CAD build for the part. Positions are in the model's coordinates, mm. Round coordinates to 2 decimals unless told otherwise and drop trailing zeros. Write each loop counter-clockwise with the first axis right and the second up, starting at its lowest first coordinate (ties: lowest second). Pieces come first, ordered by that corner, then holes. Notation, with made-up numbers: (66, -32) - (87, -32) arc R26 cw to (87, -15) - close; hole circle Ø11 at (88.25, -27). An arc over 180 degrees is marked (long way). Put each result on its own line as item: value. Start each with the question number.
Item 1: Pin check, flat tips, straight feed: pin 1 Ø2.5 at (y, z) = (-15, 120) entering from -X; pin 2 Ø5 at (x, z) = (5, 95) entering from -Y. Stop position of each tip, or through.
Item 2: Cut at A-A (x = 11). Give the cut face in (y, z), and give its area (3 significant figures).
Item 3: Drill centre lines: line 1 (X direction, y = -18.9, z = 55) (3 decimals); line 2 (X direction, y = -6.75, z = 173); line 3 (Y direction, x = 11, z = 27). Where is each one in solid material? Low to high. Write a range as from..to.
Item 4: Mould opens along X. For faces 1 (the cylindrical face through (5.473, -0.74, 191.502)), 2 (the cylindrical face through (0.74, -4.659, 18.462)), 3 (the cylindrical face through (14.397, -19.24, 121.455)) say: released by +X, released by -X, zero draft, split by the parting line, or undercut.
Item 5: Cut at B-B (z = 106). Give the cut face in (x, y), and give its area (3 significant figures).
Item 6: Cut at C-C (z = 76.5). Give the cut face in (x, y), and give its area (3 significant figures).
```python
from build123d import *

# Parameters (mm, degrees)
SKETCH_1_W          = 20
SKETCH_1_H          = 20
SKETCH_1_W_2        = 17
SKETCH_1_H_2        = 17
EXTRUDE_1_DEPTH     = 205
SKETCH_2_R          = 2.7
SKETCH_2_R_2        = 1.575
CUT_EXTRUDE_1_DEPTH = 207.942020866
SKETCH_3_R          = 1.575
CUT_EXTRUDE_2_DEPTH = 207.942020866


with BuildPart() as part:
    # 草图1 → 拉伸-薄壁1 (new body)
    with BuildSketch(Plane.XY):
        with Locations((10, -10)):
            Rectangle(SKETCH_1_W, SKETCH_1_H)
        with Locations((10, -10)):
            Rectangle(SKETCH_1_W_2, SKETCH_1_H_2, mode=Mode.SUBTRACT)
    extrude(amount=EXTRUDE_1_DEPTH)

    # 草图2 → 切除-拉伸1 (cut, through all)
    with BuildSketch(Plane.ZY):
        with Locations(Location((106, -15, 0), (0, 0, 270))):
            Circle(SKETCH_2_R)
        with Locations(Location((180, -5, 0), (0, 0, 270))):
            Circle(SKETCH_2_R_2)
        with Locations(Location((180, -15, 0), (0, 0, 270))):
            Circle(SKETCH_2_R_2)
        with Locations(Location((170, -15, 0), (0, 0, 270))):
            Circle(SKETCH_2_R_2)
        with Locations(Location((170, -5, 0), (0, 0, 270))):
            Circle(SKETCH_2_R_2)
        with Locations(Location((120, -5, 0), (0, 0, 270))):
            Circle(SKETCH_2_R_2)
        with Locations(Location((130, -5, 0), (0, 0, 270))):
            Circle(SKETCH_2_R_2)
        with Locations(Location((120, -15, 0), (0, 0, 270))):
            Circle(SKETCH_2_R_2)
        with Locations(Location((130, -15, 0), (0, 0, 270))):
            Circle(SKETCH_2_R_2)
        with Locations(Location((70, -5, 0), (0, 0, 270))):
            Circle(SKETCH_2_R_2)
        with Locations(Location((80, -5, 0), (0, 0, 270))):
            Circle(SKETCH_2_R_2)
        with Locations(Location((70, -15, 0), (0, 0, 270))):
            Circle(SKETCH_2_R_2)
        with Locations(Location((80, -15, 0), (0, 0, 270))):
            Circle(SKETCH_2_R_2)
        with Locations(Location((20, -5, 0), (0, 0, 270))):
            Circle(SKETCH_2_R_2)
        with Locations(Location((30, -5, 0), (0, 0, 270))):
            Circle(SKETCH_2_R_2)
        with Locations(Location((20, -15, 0), (0, 0, 270))):
            Circle(SKETCH_2_R_2)
        with Locations(Location((30, -15, 0), (0, 0, 270))):
            Circle(SKETCH_2_R_2)
    extrude(amount=-CUT_EXTRUDE_1_DEPTH, mode=Mode.SUBTRACT)

    # 草图3 → 切除-拉伸2 (cut, through all)
    with BuildSketch(Plane(origin=(0, 0, 0), x_dir=(1, 0, 0), z_dir=(0, 1, 0))):
        with Locations(Location((5, -5, 0), (0, 0, 270))):
            Circle(SKETCH_3_R)
        with Locations(Location((15, -5, 0), (0, 0, 90))):
            Circle(SKETCH_3_R)
        with Locations(Location((15, -15, 0), (0, 0, 270))):
            Circle(SKETCH_3_R)
        with Locations(Location((5, -15, 0), (0, 0, 90))):
            Circle(SKETCH_3_R)
        with Locations(Location((5, -190, 0), (0, 0, 270))):
            Circle(SKETCH_3_R)
        with Locations(Location((15, -190, 0), (0, 0, 90))):
            Circle(SKETCH_3_R)
        with Locations(Location((15, -200, 0), (0, 0, 270))):
            Circle(SKETCH_3_R)
        with Locations(Location((5, -200, 0), (0, 0, 90))):
            Circle(SKETCH_3_R)
        with Locations(Location((5, -150, 0), (0, 0, 270))):
            Circle(SKETCH_3_R)
        with Locations(Location((15, -150, 0), (0, 0, 90))):
            Circle(SKETCH_3_R)
        with Locations(Location((5, -160, 0), (0, 0, 90))):
            Circle(SKETCH_3_R)
        with Locations(Location((15, -160, 0), (0, 0, 270))):
            Circle(SKETCH_3_R)
        with Locations(Location((5, -110, 0), (0, 0, 270))):
            Circle(SKETCH_3_R)
        with Locations(Location((15, -110, 0), (0, 0, 90))):
            Circle(SKETCH_3_R)
        with Locations(Location((5, -120, 0), (0, 0, 90))):
            Circle(SKETCH_3_R)
        with Locations(Location((15, -120, 0), (0, 0, 270))):
            Circle(SKETCH_3_R)
        with Locations(Location((15, -85, 0), (0, 0, 90))):
            Circle(SKETCH_3_R)
        with Locations(Location((5, -85, 0), (0, 0, 270))):
            Circle(SKETCH_3_R)
        with Locations(Location((15, -95, 0), (0, 0, 270))):
            Circle(SKETCH_3_R)
        with Locations(Location((5, -95, 0), (0, 0, 90))):
            Circle(SKETCH_3_R)
        with Locations(Location((15, -45, 0), (0, 0, 90))):
            Circle(SKETCH_3_R)
        with Locations(Location((5, -45, 0), (0, 0, 270))):
            Circle(SKETCH_3_R)
        with Locations(Location((15, -55, 0), (0, 0, 270))):
            Circle(SKETCH_3_R)
        with Locations(Location((5, -55, 0), (0, 0, 90))):
            Circle(SKETCH_3_R)
    extrude(amount=-CUT_EXTRUDE_2_DEPTH, mode=Mode.SUBTRACT)


solid = part.part
```
Output values:
1. pin 1: through
1. pin 2: y = -20
2. outline: (-20, 0) - (-18.5, 0) - (-18.5, 205) - (-20, 205) - close; (-1.5, 0) - (0, 0) - (0, 205) - (-1.5, 205) - close
2. area: 615 mm2
3. line 1: 0..3.425, 6.575..13.425, 16.575..20
3. line 2: 0..1.5, 18.5..20
3. line 3: -20..-18.5, -1.5..0
4. face 1: undercut
4. face 2: zero draft
4. face 3: undercut
5. outline: (0, -20) - (20, -20) - (20, -17.7) - (18.5, -17.7) - (18.5, -18.5) - (1.5, -18.5) - (1.5, -17.7) - (0, -17.7) - close; (0, -12.3) - (1.5, -12.3) - (1.5, -1.5) - (18.5, -1.5) - (18.5, -12.3) - (20, -12.3) - (20, 0) - (0, 0) - close
5. area: 94.8 mm2
6. outline: (0, -20) - (20, -20) - (20, 0) - (0, 0) - close; hole (1.5, -18.5) - (18.5, -18.5) - (18.5, -1.5) - (1.5, -1.5) - close
6. area: 111 mm2
